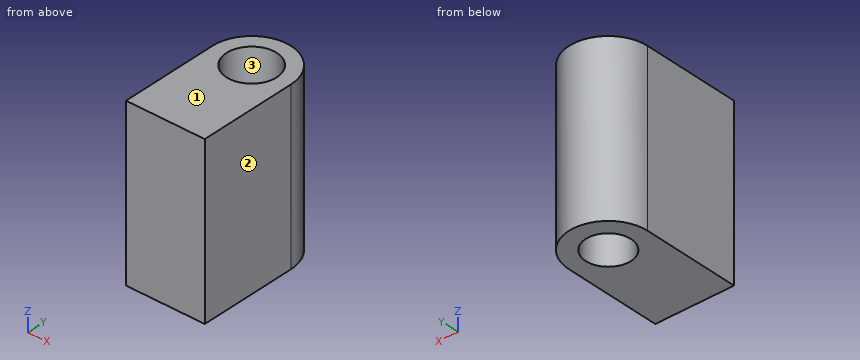
from build123d import *

# Parameters (mm, degrees)
SKETCH1_R           = 4
SKETCH1_R_2         = 2.3
BOSS_EXTRUDE1_DEPTH = 6
SKETCH2_R           = 4
SKETCH2_R_2         = 2.55
BOSS_EXTRUDE2_DEPTH = 11
SKETCH3_R           = 2.55
BOSS_EXTRUDE3_DEPTH = 17


with BuildPart() as part:
    # Sketch1 → Boss-Extrude1 (new body)
    with BuildSketch(Plane.XY):
        Circle(SKETCH1_R)
        Circle(SKETCH1_R_2, mode=Mode.SUBTRACT)
    extrude(amount=BOSS_EXTRUDE1_DEPTH)

    # Sketch2 → Boss-Extrude2 (add)
    with BuildSketch(Plane.XY.offset(6)):
        Circle(SKETCH2_R)
        Circle(SKETCH2_R_2, mode=Mode.SUBTRACT)
    extrude(amount=BOSS_EXTRUDE2_DEPTH)

    # Sketch3 → Boss-Extrude3 (add)
    with BuildSketch(Plane(origin=(0, 0, 0), x_dir=(-1, 0, 0), z_dir=(0, 0, -1))):
        with BuildLine():
            Line((-4, 0), (-4, -10))
            Line((-4, -10), (4, -10))
            Line((4, -10), (4, 0))
            ThreePointArc((4, 0), (0, 4), (-4, 0))
        make_face()
        with Locations(Location((0, 0, 0), (0, 0, 180))):
            Circle(SKETCH3_R, mode=Mode.SUBTRACT)
    extrude(amount=-BOSS_EXTRUDE3_DEPTH)


solid = part.part
The listing builds one solid part. Answer for the finished solid, in the listing's coordinates (mm). Face numbers are marked on the shaded views. Give positions to 0.01 mm unless a question says otherwise; leave off trailing zeros. Write each loop counter-clockwise with the first axis right and the second up, starting at its lowest first coordinate (ties: lowest second). Pieces come first, ordered by that corner, then holes.
Item 1: Find the intervals of material crossed by line 1 along Y through (x, z) = (0, 12.75); line 2 along Y through (x, z) = (0, 2.5); line 3 along X through (y, z) = (-0.25, 8.25), in increasing order.
Item 2: Section D-D, the plane z = 8.25 is taken. Write down the section's boundary in (x, y), plus the area to 3 significant figures.
Item 3: Section B-B, the plane z = 5.75 is taken. Write down the section's boundary in (x, y).
Item 4: Determine the mould class of the marked faces 1, 2 and 3 for opening direction X: released by +X, released by -X, zero draft, split by the parting line, or undercut.
Item 5: Section C-C, the plane y = 1.75 is taken. Write down the section's boundary in (x, z).
Item 6: Section A-A, the plane x = 0 is taken. Write down the section's boundary in (y, z), plus the area to 3 significant figures.
Completed:
1. line 1: y = -10 to -2.55, 2.55 to 4
1. line 2: y = -10 to -2.3, 2.3 to 4
1. line 3: x = -4 to -2.54, 2.54 to 4
2. outline: (-4, -10) - (4, -10) - (4, 0) arc R4 ccw to (-4, 0) - close; hole circle Ø5.1 at (0, 0)
2. area: 84.7 mm2
3. outline: (-4, -10) - (4, -10) - (4, 0) arc R4 ccw to (-4, 0) - close; hole circle Ø4.6 at (0, 0)
4. face 1: zero draft
4. face 2: released by +X
4. face 3: undercut
5. outline: (-3.6, 0) - (-1.49, 0) - (-1.49, 6) - (-1.85, 6) - (-1.85, 17) - (-3.6, 17) - close; (1.49, 0) - (3.6, 0) - (3.6, 17) - (1.85, 17) - (1.85, 6) - (1.49, 6) - close
6. outline: (-10, 0) - (-2.3, 0) - (-2.3, 6) - (-2.55, 6) - (-2.55, 17) - (-10, 17) - close; (2.3, 0) - (4, 0) - (4, 17) - (2.55, 17) - (2.55, 6) - (2.3, 6) - close
6. area: 154 mm2
